Source: CAD feature listing. Evaluate the final solid. Frame: model axes, mm. A direction names the side the tool comes from. Round coordinates to 2 decimals unless told otherwise and drop trailing zeros. Loops run counter-clockwise (first coordinate to the right, second up) from the corner with the lowest first, then second, coordinate; pieces in that order, holes last. Notation, with made-up numbers: M 49.25,-9 L 89.25,-9 A33 cw 89.25,29 Z; hole C 8,-9 d11. An arc over 180 degrees is marked long. Write each question's results on one line, items separated by ' | '. Start each with the question number.
1. Contact query for flat-ended pins moving along their axis: pin 1 Ø1.1 at (x, z) = (-142.5, 56.5) entering from +Y; pin 2 Ø3 at (y, z) = (18, 73) entering from -X; pin 3 Ø0.8 at (y, z) = (21.5, 104.5) entering from -X. Output: stop coordinate, or through.
2. Ray query, line 1 (Z direction, x = -129, y = 19.5); line 2 (Z direction, x = -58, y = 16); line 3 (X direction, y = 19.25, z = 68). Return the intervals inside material, ascending.
3. Set-up query: faces 4 (the flat face through (-73, 20, -2)), 5 (the flat face through (-39, 12, 71)), 6 (the flat face through (-3.5, 12, 33)). Return all of +Z, -Z, +X, -X, +Y, -Y with unobstructed straight access to the full face (end or side cutting, diameter ignored); none if empty.
4. Draft query along Z for faces 1 (the flat face through (-143, 2, 59)), 2 (the flat face through (-100.89, 20.07, 89.37)), 3 (the flat face through (-74, 13, -3.5)). Return one class per face: released by +Z, released by -Z, zero draft, split by the parting line, or undercut.
5. Section C-C on z = 47. Output: boundary loops of the cut face in (x, y).
6. Section D-D on y = 20. Output: boundary loops of the cut face in (x, z).
7. Section B-B on x = -132. Output: boundary loops of the cut face in (y, z).
8. Section A-A on y = 6. Output: boundary loops of the cut face in (x, z).
from build123d import *

# Parameters (mm, degrees)
BOSS_EXTRUDE1_DEPTH = 25
CUT_EXTRUDE1_DEPTH  = 22
SKETCH7_W           = 4
SKETCH7_H           = 106
CUT_EXTRUDE2_DEPTH  = 22
SKETCH8_W           = 3
SKETCH8_H           = 106
CUT_EXTRUDE3_DEPTH  = 1.5
SKETCH9_W           = 3
SKETCH9_H           = 23.5
CUT_EXTRUDE4_DEPTH  = 1.5
CUT_EXTRUDE5_DEPTH  = 10
BOSS_EXTRUDE2_DEPTH = 13.5
BOSS_EXTRUDE3_DEPTH = 107.5


with BuildPart() as part:
    # PCB → Boss-Extrude1 (new body)
    with BuildSketch(Plane(origin=(0, 0, 0), x_dir=(1, 0, 0), z_dir=(0, 1, 0))):
        Polygon((-3.5, 3.5), (-3.5, -71), (-75.5, -71), (-75.5, -75.988917258), (-125.036460317, -105.5), (-142, -105.5), (-143, -105.5), (-143, 3.5), (-142, 3.5), align=None)
    extrude(amount=BOSS_EXTRUDE1_DEPTH)

    # Sketch4 → Cut-Extrude1 (cut)
    with BuildSketch(Plane(origin=(0, 25, 0), x_dir=(1, 0, 0), z_dir=(0, 1, 0))):
        Polygon((-6.5, 0.5), (-140, 0.5), (-140, -102.5), (-125.862351474, -102.5), (-78.5, -74.284131037), (-78.5, -68), (-6.5, -68), align=None)
    extrude(amount=-CUT_EXTRUDE1_DEPTH, mode=Mode.SUBTRACT)

    # Sketch7 → Cut-Extrude2 (cut)
    with BuildSketch(Plane(origin=(0, 25, 0), x_dir=(1, 0, 0), z_dir=(0, 1, 0))):
        with Locations((-141, -49.5)):
            Rectangle(SKETCH7_W, SKETCH7_H)
    extrude(amount=-CUT_EXTRUDE2_DEPTH, mode=Mode.SUBTRACT)

    # Sketch8 → Cut-Extrude3 (cut)
    with BuildSketch(Plane(origin=(0, 3, 0), x_dir=(1, 0, 0), z_dir=(0, 1, 0))):
        with Locations((-140.5, -49.5)):
            Rectangle(SKETCH8_W, SKETCH8_H)
    extrude(amount=-CUT_EXTRUDE3_DEPTH, mode=Mode.SUBTRACT)

    # Sketch9 → Cut-Extrude4 (cut)
    with BuildSketch(Plane(origin=(0, 0, 102.5), x_dir=(-1, 0, 0), z_dir=(0, 0, -1))):
        with Locations((140.5, 13.25)):
            Rectangle(SKETCH9_W, SKETCH9_H)
    extrude(amount=-CUT_EXTRUDE4_DEPTH, mode=Mode.SUBTRACT)

    # Sketch10 → Cut-Extrude5 (cut)
    with BuildSketch(Plane(origin=(0, 25, 0), x_dir=(1, 0, 0), z_dir=(0, 1, 0))):
        Polygon((-138, -105.5), (-143, -105.5), (-143, -102.5), (-142, -102.5), (-142, -104), (-139, -104), (-139, -102.5), (-125.862351474, -102.5), (-78.5, -74.284131037), (-78.5, -68), (-6.5, -68), (-6.5, 0.5), (-139, 0.5), (-139, 2), (-5, 2), (-5, -69.5), (-77, -69.5), (-77, -75.136524148), (-125.449405895, -104), (-138, -104), align=None)
    extrude(amount=-CUT_EXTRUDE5_DEPTH, mode=Mode.SUBTRACT)

    # Sketch11 → Boss-Extrude2 (add)
    with BuildSketch(Plane(origin=(0, 1.5, 0), x_dir=(1, 0, 0), z_dir=(0, 1, 0))):
        Polygon((-142, -102.5), (-139, -104), (-142, -104), align=None)
    extrude(amount=BOSS_EXTRUDE2_DEPTH)

    # Sketch12 → Boss-Extrude3 (add)
    with BuildSketch(Plane(origin=(0, 0, -3.5), x_dir=(-1, 0, 0), z_dir=(0, 0, -1))):
        Polygon((139, 1.5), (142, 3), (142, 1.5), align=None)
    extrude(amount=-BOSS_EXTRUDE3_DEPTH)


solid = part.part
Taken from the geometry:
1) pin 1: y = 3 | pin 2: x = -77 | pin 3: x = -138
2) line 1: -3.5 to -2, 104 to 105.5 | line 2: -3.5 to -2, 69.5 to 71 | line 3: -5 to -3.5
3) face 4: -X, +Y | face 5: +Z, +X, +Y, -Y | face 6: +Z, -Z, +X, +Y, -Y
4) face 1: zero draft | face 2: undercut | face 3: released by -Z
5) outline: M -143,0 L -3.5,0 L -3.5,25 L -5,25 L -5,15 L -6.5,15 L -6.5,3 L -139,3 L -139,1.5 L -142,3 L -143,3 Z
6) outline: M -139,-3.5 L -3.5,-3.5 L -3.5,71 L -75.5,71 L -75.5,75.99 L -125.04,105.5 L -138,105.5 L -138,104 L -125.45,104 L -77,75.14 L -77,69.5 L -5,69.5 L -5,-2 L -139,-2 Z
7) outline: M 0,-3.5 L 25,-3.5 L 25,-2 L 15,-2 L 15,-0.5 L 3,-0.5 L 3,102.5 L 15,102.5 L 15,104 L 25,104 L 25,105.5 L 0,105.5 Z
8) outline: M -143,102.5 L -142,102.5 L -139,104 L -139,102.5 L -125.86,102.5 L -78.5,74.28 L -78.5,68 L -6.5,68 L -6.5,-0.5 L -139,-0.5 L -139,-3.5 L -3.5,-3.5 L -3.5,71 L -75.5,71 L -75.5,75.99 L -125.04,105.5 L -143,105.5 Z
